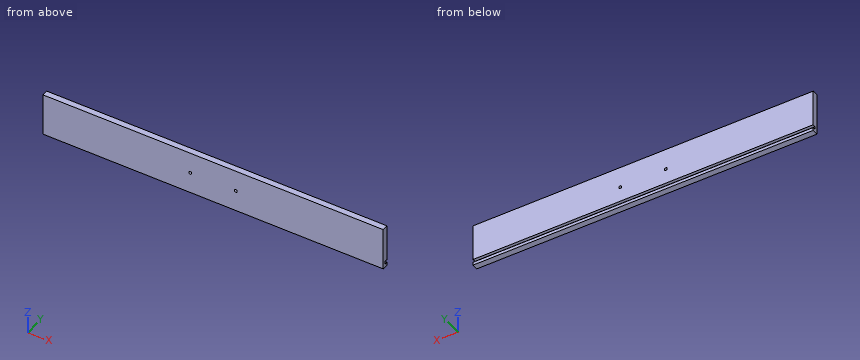
```python
from build123d import *

# Parameters (mm, degrees)
PAD_DEPTH   = 717.5
SKETCH003_R = 3
HOLE_DEPTH  = 12.701


with BuildPart() as part:
    # Sketch → Pad (new body)
    with BuildSketch(Plane.YZ):
        Polygon((0, 0), (12.7, 0), (12.7, 6.35), (6.35, 6.35), (6.35, 12.7), (12.7, 12.7), (12.7, 88.9), (0, 88.9), align=None)
    extrude(amount=PAD_DEPTH)

    # Sketch003 → Hole (cut, through all)
    with BuildSketch(Plane(origin=(0, 0, 0), x_dir=(0, 0, -1), z_dir=(0, -1, 0))):
        with Locations((-44.45, 310.75)):
            Circle(SKETCH003_R)
        with Locations((-44.45, 406.75)):
            Circle(SKETCH003_R)
    extrude(amount=-HOLE_DEPTH, mode=Mode.SUBTRACT)


solid = part.part
```
Geometry: final body of the model. Coordinates: model frame, mm. Round coordinates to 2 decimals unless told otherwise and drop trailing zeros. Write each loop counter-clockwise with the first axis right and the second up, starting at its lowest first coordinate (ties: lowest second). Pieces come first, ordered by that corner, then holes. Notation, with made-up numbers: M 82.25,-0.5 L 110.25,-0.5 A21 ccw 110.25,18.5 Z; hole C 15.25,-14 d2. An arc over 180 degrees is marked long. Answer in a Markdown table with one row per item. Add a question column.
(1) Cut plane A-A, the plane y = 8.75. Return the cut outline in (x, z).
(2) Cut plane B-B, the plane x = 140.5. Return the cut outline in (y, z), then the cut area to 3 significant figures.
(3) Contact query for a flat-ended pin moving along its axis: pin 1 (3 mm diameter, centred on x = 485, z = 8.5, fed in from +Y). Output: stop coordinate, or through.
(4) Ray query, L1, parallel to X at y = 8.5, z = 44.45; L2, parallel to Z at x = 406.75, y = 7; L3, parallel to Z at x = 468, y = 12.25. Return the intervals inside material, ascending.
Established:
| question | item | result |
|---|---|---|
| 1 | outline | M 0,0 L 717.5,0 L 717.5,6.35 L 0,6.35 Z; M 0,12.7 L 717.5,12.7 L 717.5,88.9 L 0,88.9 Z; hole C 310.75,44.45 d6; hole C 406.75,44.45 d6 |
| 2 | outline | M 0,0 L 12.7,0 L 12.7,6.35 L 6.35,6.35 L 6.35,12.7 L 12.7,12.7 L 12.7,88.9 L 0,88.9 Z |
| 2 | area | 1,090 mm² |
| 3 | pin 1 | y = 6.35 |
| 4 | L1 | 0 to 307.75, 313.75 to 403.75, 409.75 to 717.5 |
| 4 | L2 | 0 to 6.35, 12.7 to 41.45, 47.45 to 88.9 |
| 4 | L3 | 0 to 6.35, 12.7 to 88.9 |
